The listing builds one solid part. Answer for the finished solid, in the listing's coordinates (mm). Face numbers are marked on the shaded views. A direction names the side the tool comes from. Give positions to 0.01 mm unless a question says otherwise; leave off trailing zeros. Loops run counter-clockwise (first coordinate to the right, second up) from the corner with the lowest first, then second, coordinate; pieces in that order, holes last. Notation, with made-up numbers: M 35,81.25 L 66,81.25 A20 ccw 66,89.25 Z; hole C 35,25.25 d8. An arc over 180 degrees is marked long. One line per item, written item: value. Start each with the question number.
Q1. A flat-ended cylindrical pin translates along its axis: pin 1 (16.5 mm diameter, centred on x = 381, z = 0, fed in from +Y). Find the tip coordinate at first contact, or state that the pin passes through.
Q2. A cutting plane is placed at A-A, the plane y = 9. Determine the outline of the cut face in (x, z).
Q3. A cutting plane is placed at C-C, the plane x = 155.5. Determine the outline of the cut face in (y, z), and give its area (3 significant figures).
Q4. For the marked faces 1 and 2, determine the directions among +Z, -Z, +X, -X, +Y, -Y from which every point of the face is accessible in a straight line to the end or side of a thin tool.
Q5. A cutting plane is placed at D-D, the plane z = 0. Determine the outline of the cut face in (x, y).
Q6. Consider L1, parallel to Z at x = 381, y = 41; L2, parallel to Y at x = 51.5, z = -3. Determine where each line is inside the solid, lowest interval first.
Q7. The mould has two halves that part along Y. Classify the marked faces 3, 4, 5 and 6: +Y half, -Y half, draft (parallel to the pull), parting line (faces both ways), or undercut.
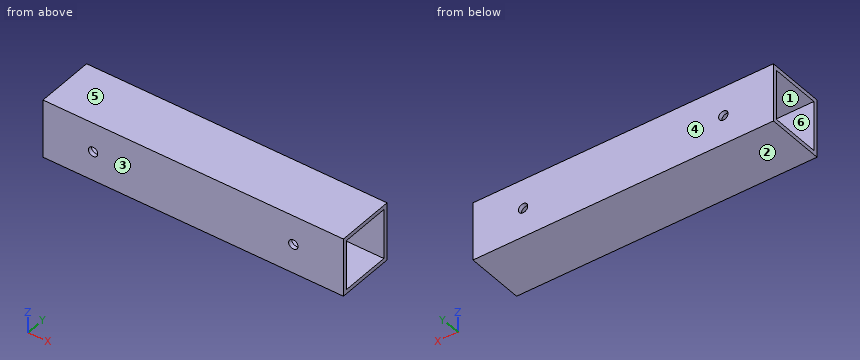
from build123d import *

# Parameters (mm, degrees)
F0_W     = 88.9
F0_H     = 88.9
F0_W_2   = 76.2
F0_H_2   = 76.2
F1_DEPTH = 457.2
F2_R     = 7.14375
F3_DEPTH = 88.901


with BuildPart() as f1:
    # F0 (on Right) → F1 (new body)
    with BuildSketch(Plane.YZ):
        Rectangle(F0_W, F0_H)
        Rectangle(F0_W_2, F0_H_2, mode=Mode.SUBTRACT)
    extrude(amount=F1_DEPTH)

    # F2 (on face) → F3 (cut, through all)
    with BuildSketch(Plane.XZ.offset(44.45)):
        with Locations((381, 0)):
            Circle(F2_R)
        with Locations((76.2, 0)):
            Circle(F2_R)
    extrude(amount=-F3_DEPTH, mode=Mode.SUBTRACT)


solid = f1.part
Answer block:
1. pin 1: y = 44.45
2. outline: M 0,-44.45 L 457.2,-44.45 L 457.2,-38.1 L 0,-38.1 Z; M 0,38.1 L 457.2,38.1 L 457.2,44.45 L 0,44.45 Z
3. outline: M -44.45,-44.45 L 44.45,-44.45 L 44.45,44.45 L -44.45,44.45 Z; hole M -38.1,-38.1 L 38.1,-38.1 L 38.1,38.1 L -38.1,38.1 Z
3. area: 2,100 mm^2
4. face 1: +X, -X
4. face 2: -Z, +X, -X, +Y, -Y
5. outline: M 0,-44.45 L 69.06,-44.45 L 69.06,-38.1 L 0,-38.1 Z; M 0,38.1 L 69.06,38.1 L 69.06,44.45 L 0,44.45 Z; M 83.34,-44.45 L 373.86,-44.45 L 373.86,-38.1 L 83.34,-38.1 Z; M 83.34,38.1 L 373.86,38.1 L 373.86,44.45 L 83.34,44.45 Z; M 388.14,-44.45 L 457.2,-44.45 L 457.2,-38.1 L 388.14,-38.1 Z; M 388.14,38.1 L 457.2,38.1 L 457.2,44.45 L 388.14,44.45 Z
6. L1: -44.45 to -7.14, 7.14 to 44.45
6. L2: -44.45 to -38.1, 38.1 to 44.45
7. face 3: -Y half
7. face 4: +Y half
7. face 5: draft
7. face 6: undercut
